```python
from build123d import *

# Parameters (mm, degrees)
F0_W      = 99.28
F0_H      = 99.28
F1_DEPTH  = 5
F2_R      = 9.975
F3_DEPTH  = 50.12
F4_R      = 6.97414
F5_DEPTH  = 45
F6_W      = 10.15
F6_H      = 33.35
F7_DEPTH  = 51.54
F8_W      = 19.84
F8_H      = 17.26
F9_DEPTH  = 30.101
F10_R     = 1.715
F11_DEPTH = 30.101
F12_W     = 99.28
F12_H     = 26.759172
F13_DEPTH = 55.121
F14_W     = 25.082288
F14_H     = 72.520828
F15_DEPTH = 55.121
F16_W     = 74.197712
F16_H     = 22.137212
F17_DEPTH = 55.121
F18_R     = 1.715
F19_DEPTH = 30.101
F20_W     = 4.45
F20_H     = 0.8
F21_DEPTH = 55.121
F22_R     = 1.72
F23_DEPTH = 55.121
F24_W     = 50.383616
F24_H     = 56.672631
F25_DEPTH = 74.198713


with BuildPart() as f1:
    # F0 (on Top) → F1 (new body)
    with BuildSketch(Plane.XY):
        with Locations((1.248532, -12.53785)):
            Rectangle(F0_W, F0_H)
    extrude(amount=F1_DEPTH)

    # F2 (on face) → F3 (join)
    with BuildSketch(Plane(origin=(0, 0, 0), x_dir=(1, 0, 0), z_dir=(0, 0, -1))):
        with Locations((0, 12.20285)):
            Circle(F2_R)
    extrude(amount=F3_DEPTH)

    # F4 (on face) → F5 (cut)
    with BuildSketch(Plane(origin=(0, 0, -50.12), x_dir=(1, 0, 0), z_dir=(0, 0, -1))):
        with Locations((0, 12.20285)):
            Circle(F4_R)
    extrude(amount=-F5_DEPTH, mode=Mode.SUBTRACT)

    # F6 (on face) → F7 (join)
    with BuildSketch(Plane.XY.offset(5)):
        with Locations((-23.366468, -12.46285)):
            Rectangle(F6_W, F6_H)
    extrude(amount=F7_DEPTH)

    # F8 (on face) → F9 (cut, through all)
    with BuildSketch(Plane.YZ.offset(-18.291468)):
        with Locations((-12.51785, 47.91)):
            Rectangle(F8_W, F8_H)
    extrude(amount=-F9_DEPTH, mode=Mode.SUBTRACT)

    # F10 (on face) → F11 (cut, through all)
    with BuildSketch(Plane.YZ.offset(-18.291468)):
        with Locations((-25.66285, 52.125)):
            Circle(F10_R)
        with Locations((-25.66285, 47.205)):
            Circle(F10_R)
    extrude(amount=-F11_DEPTH, mode=Mode.SUBTRACT)

    # F12 (on face) → F13 (cut, through all)
    with BuildSketch(Plane.XY.offset(5)):
        with Locations((1.248532, 23.722564)):
            Rectangle(F12_W, F12_H)
    extrude(amount=-F13_DEPTH, mode=Mode.SUBTRACT)

    # F14 (on face) → F15 (cut, through all)
    with BuildSketch(Plane.XY.offset(5)):
        with Locations((38.347388, -25.917436)):
            Rectangle(F14_W, F14_H)
    extrude(amount=-F15_DEPTH, mode=Mode.SUBTRACT)

    # F16 (on face) → F17 (cut, through all)
    with BuildSketch(Plane.XY.offset(5)):
        with Locations((-11.292612, -51.109244)):
            Rectangle(F16_W, F16_H)
    extrude(amount=-F17_DEPTH, mode=Mode.SUBTRACT)

    # F18 (on face) → F19 (cut, through all)
    with BuildSketch(Plane.YZ.offset(-18.291468)):
        with Locations((0.73715, 52.125)):
            Circle(F18_R)
        with Locations((0.73715, 47.205)):
            Circle(F18_R)
    extrude(amount=-F19_DEPTH, mode=Mode.SUBTRACT)

    # F20 (on face) → F21 (cut, through all)
    with BuildSketch(Plane.XY.offset(5)):
        with Locations((-16.306812, -38.074275)):
            Rectangle(F20_W, F20_H)
        with Locations((-16.306812, 6.925725)):
            Rectangle(F20_W, F20_H)
        with Locations((9.693188, -38.074275)):
            Rectangle(F20_W, F20_H)
        with Locations((9.693188, 6.925725)):
            Rectangle(F20_W, F20_H)
    extrude(amount=-F21_DEPTH, mode=Mode.SUBTRACT)

    # F22 (on face) → F23 (cut, through all)
    with BuildSketch(Plane.XY.offset(5)):
        with Locations((-43.671468, 5.622978)):
            Circle(F22_R)
        with Locations((-43.671468, -35.377022)):
            Circle(F22_R)
        with Locations((21.328532, 5.622978)):
            Circle(F22_R)
        with Locations((21.328532, -35.377022)):
            Circle(F22_R)
    extrude(amount=-F23_DEPTH, mode=Mode.SUBTRACT)

    # F24 (on face) → F25 (cut, through all)
    with BuildSketch(Plane.YZ.offset(25.806244)):
        with Locations((-14.84883, -25.836315)):
            Rectangle(F24_W, F24_H)
    extrude(amount=-F25_DEPTH, mode=Mode.SUBTRACT)


solid = f1.part
```
Source: CAD feature listing. Evaluate the final solid. Frame: model axes, mm. A direction names the side the tool comes from. Give positions to 0.01 mm unless a question says otherwise; leave off trailing zeros. Loops run counter-clockwise (first coordinate to the right, second up) from the corner with the lowest first, then second, coordinate; pieces in that order, holes last. Notation, with made-up numbers: (44.5, 69) -> (60.5, 69) arc R15 ccw to (60.5, 91) -> close; hole circle Ø11 at (37, 2). An arc over 180 degrees is marked (long way). Use a Markdown table: item, result. Add a question column.
(1) Access query for faces 1 (the face through (-23, -13, 39.28)), 2 (the face through (-23, -29.138, 30)), 3 (the face through (-18.291, -13, 25)). Directions: +Z, -Z, +X, -X, +Y, -Y. A direction counts if a zero-diameter tool reaches every point of the face in a straight line with its end or side. Return the directions, or none.
(2) Section query B-B (y = -12). Output: boundary loops of the cut face in (x, z).
(3) Section query C-C (x = -16.5). Output: boundary loops of the cut face in (y, z).
(4) Ray query, line 1 (X direction, y = -21.5, z = 33.5); line 2 (Z direction, x = 12.5, y = 0.5); line 3 (Y direction, x = -22, z = 28). Return the intervals inside material, ascending.
(5) Section query A-A (z = 43.5). Output: boundary loops of the cut face in (x, y).
(6) Section query D-D (x = -27.5). Output: boundary loops of the cut face in (y, z) (3 decimals).
(7) Pull-direction query (Z, two-part tool) for faces 4 (the face through (-16, -37.674, 4)), 5 (the face through (-23.3, -24.1, 46.5)), 6 (the face through (-12, -14, 5)); classes: +Z half, -Z half, draft (parallel to the pull), parting line (faces both ways), or undercut.
(8) First-contact query: pin 1 Ø12 at (y, z) = (-2, 34.5) entering from +X; pin 2 Ø10 at (x, y) = (-28, -10.5) entering from +Z; pin 3 Ø4.5 at (y, z) = (0.74, 47.2) entering from -X. Flat tips, straight axial feed; report the tip coordinate or a pass-through.
Checked values:
| question | item | result |
|---|---|---|
| 1 | face 1 | +Z, +X, -X |
| 1 | face 2 | +Z, +X, -X, -Y |
| 1 | face 3 | +Z, +X, +Y, -Y |
| 2 | outline | (-48.39, 2.5) -> (25.81, 2.5) -> (25.81, 5) -> (-18.29, 5) -> (-18.29, 39.28) -> (-28.44, 39.28) -> (-28.44, 5) -> (-48.39, 5) -> close |
| 3 | outline | (-40.04, 2.5) -> (-38.47, 2.5) -> (-38.47, 5) -> (-40.04, 5) -> close; (-37.67, 2.5) -> (6.53, 2.5) -> (6.53, 5) -> (-37.67, 5) -> close; (7.33, 2.5) -> (10.34, 2.5) -> (10.34, 5) -> (7.33, 5) -> close |
| 4 | line 1 | -28.44 to -18.29 |
| 4 | line 2 | 2.5 to 5 |
| 4 | line 3 | -29.14 to 4.21 |
| 5 | outline | (-28.44, -29.14) -> (-18.29, -29.14) -> (-18.29, -22.44) -> (-28.44, -22.44) -> close; (-28.44, -2.6) -> (-18.29, -2.6) -> (-18.29, 4.21) -> (-28.44, 4.21) -> close |
| 6 | outline | (-40.041, 2.5) -> (10.343, 2.5) -> (10.343, 5) -> (4.212, 5) -> (4.212, 56.54) -> (-2.598, 56.54) -> (-2.598, 39.28) -> (-22.438, 39.28) -> (-22.438, 56.54) -> (-29.138, 56.54) -> (-29.138, 5) -> (-40.041, 5) -> close; hole circle Ø3.43 at (-25.663, 47.205); hole circle Ø3.43 at (-25.663, 52.125); hole circle Ø3.43 at (0.737, 47.205); hole circle Ø3.43 at (0.737, 52.125) |
| 7 | face 4 | draft |
| 7 | face 5 | undercut |
| 7 | face 6 | +Z half |
| 8 | pin 1 | x = -18.29 |
| 8 | pin 2 | z = 39.28 |
| 8 | pin 3 | x = -28.44 |
